Autodesk Inventor part; units mm, degrees
ref_plane "YZ Plane" through (0, 0, 0) normal (1, 0, 0) x (0, 1, 0)
ref_plane "XZ Plane" through (0, 0, 0) normal (0, 1, 0) x (-1, 0, 0)
ref_plane "XY Plane" through (0, 0, 0) normal (0, 0, 1) x (1, 0, 0)
sketch "Sketch3" plane through (0, 0, 0) normal (0, 1, 0) x (-1, 0, 0)
  line L0 (0, 0) -> (0, 43)
  line L1 (-11, 0) -> (-12, 0)
  line L2 (-12, 0) -> (-12, 28)
  line L3 (-12, 28) -> (-21.75, 28)
  line L4 (-21.75, 28) -> (-21.75, 36.5)
  line L5 (-21.75, 36.5) -> (-18.75, 36.5)
  line L6 (-18.75, 36.5) -> (-18.75, 40)
  line L7 (-18.75, 40) -> (-21.75, 40)
  line L8 (-21.75, 40) -> (-21.75, 43)
  line L9 (-21.75, 43) -> (-17.4, 43)
  line L10 (-17.4, 43) -> (-5.5, 33.0147)
  line L11 (-5.5, 33.0147) -> (-5.5, 29.6753)
  line L12 (-5.5, 29.6753) -> (-11, 0)
  dimension "d1" = 24
  dimension "d2" = 28
  dimension "d3" = 43
  dimension "d5" = 3.5
  dimension "d6" = 43.5
  dimension "d7" = 37.5
  dimension "d8" = 34.8
  dimension "d9" = 11
  dimension "d10" = 29.6753
  dimension "d11" = 9.9853
  dimension "d12" = 22
  dimension "d14" = 10.5
  dimension "d15" = 50
  dimension "d17" = 36.5
revolve "Revolution1" add sketch "Sketch3" angle 360 about axis through (0, 0, 0) along (0, 0, 1)
chamfer "Chamfer1" distance 0.5 angle 45 2 edges at (-21.75, 0, 43) (-21.75, 0, 28)
properties part number "Nozzle" material "Steel"
Read the model definition and answer for the solid it produces. Units are mm, in the model's axes. A direction names the side the tool comes from. Give positions to 0.01 mm unless a question says otherwise; leave off trailing zeros. Write each loop counter-clockwise with the first axis right and the second up, starting at its lowest first coordinate (ties: lowest second). Pieces come first, ordered by that corner, then holes. Notation, with made-up numbers: M 57.25,68 L 113.25,68 A13 ccw 113.25,86 Z; hole C 68,58.25 d6. An arc over 180 degrees is marked long. One line per item, written item: value. Start each with the question number.
(1) Find section A-A (x = 0). Determine the outline of the cut face in (y, z).
(2) Flat-ended cylindrical pins translate along their axes: pin 1 Ø12 at (x, z) = (2, 5) entering from -Y; pin 2 Ø6 at (x, y) = (-13, 17) entering from +Z; pin 3 Ø1.5 at (y, z) = (-0.5, 13) entering from +X; pin 4 Ø13 at (x, y) = (-9, -1.5) entering from +Z. Find the tip coordinate at first contact, or state that the pin passes through.
(3) Find section C-C (z = 6.5). Determine the outline of the cut face in (x, y).
(4) Find the intervals of material crossed by line 1 (Y direction, x = 0, z = 31.4); line 2 (Z direction, x = 5, y = -18.5); line 3 (X direction, y = -4, z = 30.5), in increasing order.
(5) A tool of negligible diameter and unlimited length cuts with its end or side. For faces 4 (the flat face through (9, -9, 28)), 5 (the cylindrical face through (-2.44, 18.59, 38.27)), 6 (the flat face through (-8, -16, 43)), from which of +Z, -Z, +X, -X, +Y, -Y can it reach the whole face along a straight path? Write none if from no direction.
(6) Find section D-D (z = 17). Determine the outline of the cut face in (x, y), plus the area to 3 significant figures.
(7) Determine the mould class of faces 1 (the conical face through (-1.8, 8.09, 14.63)), 2 (the cylindrical face through (-2.831, 21.565, 32.556)), 3 (the flat face through (5, -10, 0)) for opening direction X: pulls with the +X half, pulls with the -X half, needs draft (parallel to the pull), parting line crosses it, or undercut.
Results below:
1. outline: M -21.75,28.5 L -21.25,28 L -12,28 L -12,0 L -11,0 L -5.5,29.68 L -5.5,33.01 L -17.4,43 L -21.25,43 L -21.75,42.5 L -21.75,40 L -18.75,40 L -18.75,36.5 L -21.75,36.5 Z; M 5.5,29.68 L 11,0 L 12,0 L 12,28 L 21.25,28 L 21.75,28.5 L 21.75,36.5 L 18.75,36.5 L 18.75,40 L 21.75,40 L 21.75,42.5 L 21.25,43 L 17.4,43 L 5.5,33.01 Z
2. pin 1: stops at y = -12
2. pin 2: stops at z = 43
2. pin 3: stops at x = 12
2. pin 4: stops at z = 41.51
3. outline: C 0,0 d24; hole C 0,0 d19.59
4. line 1: y = -21.75 to -5.5, 5.5 to 21.75
4. line 2: z = 28 to 36.5, 40 to 43
4. line 3: x = -21.38 to -3.77, 3.77 to 21.38
5. face 4: -Z
5. face 5: none
5. face 6: +Z, +X, -X, +Y, -Y
6. outline: C 0,0 d24; hole C 0,0 d15.7
6. area: 259 mm^2
7. face 1: undercut
7. face 2: parting line crosses it
7. face 3: needs draft
